Source: CAD feature listing. Evaluate the final solid. Frame: model axes, mm. A direction names the side the tool comes from. Coordinates: 2 decimals unless noted, no trailing zeros. Loops run counter-clockwise (first coordinate to the right, second up) from the corner with the lowest first, then second, coordinate; pieces in that order, holes last. Notation, with made-up numbers: M 81.25,-4.5 L 88.25,-4.5 A16 cw 88.25,10.5 Z; hole C -30.75,1.5 d2. An arc over 180 degrees is marked long. Write each question's results on one line, items separated by ' | '. Start each with the question number.
from build123d import *

# Parameters (mm, degrees)
BOSS_EXTRUDE1_DEPTH = 175


with BuildPart() as part:
    # Sketch1 → Boss-Extrude1 (new body, symmetric)
    with BuildSketch(Plane.XY):
        Polygon((-3.1, 10), (-3.1, 8.200660172), (-5.5, 8.200660172), (-5.5, 6.560660172), (-2.84, 3.900660172), (2.84, 3.900660172), (5.5, 6.560660172), (5.5, 8.200660172), (3.1, 8.200660172), (3.1, 10), (10, 10), (10, 3.1), (8.200660172, 3.1), (8.200660172, 5.5), (6.560660172, 5.5), (3.900660172, 2.84), (3.900660172, -2.84), (6.560660172, -5.5), (8.200660172, -5.5), (8.200660172, -3.1), (10, -3.1), (10, -10), (3.1, -10), (3.1, -8.200660172), (5.5, -8.200660172), (5.5, -6.560660172), (2.84, -3.900660172), (-2.84, -3.900660172), (-5.5, -6.560660172), (-5.5, -8.200660172), (-3.1, -8.200660172), (-3.1, -10), (-10, -10), (-10, -3.1), (-8.200660172, -3.1), (-8.200660172, -5.5), (-6.560660172, -5.5), (-3.900660172, -2.84), (-3.900660172, 2.84), (-6.560660172, 5.5), (-8.200660172, 5.5), (-8.200660172, 3.1), (-10, 3.1), (-10, 10), align=None)
    extrude(amount=BOSS_EXTRUDE1_DEPTH, both=True)


solid = part.part
Item 1: Cut plane A-A (y = 0). Output: boundary loops of the cut face in (x, z), then the cut area to 3 significant figures.
Item 2: Access query for faces 4 (the flat face through (10, 7, 2)), 5 (the flat face through (0, -3.901, 2)), 6 (the flat face through (0, 3.901, 2)), 7 (the flat face through (-7, 10, 2)), 8 (the flat face through (-3.901, 0, 2)). Directions: +Z, -Z, +X, -X, +Y, -Y. A direction counts if a zero-diameter tool reaches every point of the face in a straight line with its end or side. Return the directions, or none.
Item 3: Line query: probe 1 along Y at (x, z) = (-8, 28.5); probe 2 along Y at (x, z) = (9.25, 122.5); probe 3 along Y at (x, z) = (-3.25, 158.5). Output: solid intervals per line, ascending.
Item 4: Mould query, pull axis Y, two halves, no side actions, for faces 1 (the flat face through (7, -10, 2)), 2 (the flat face through (10, -7, 2)), 3 (the flat face through (3.901, 0, 2)). Classes: +Y half, -Y half, draft (parallel to the pull), parting line (faces both ways), or undercut.
Item 5: First-contact query: pin 1 Ø3 at (y, z) = (-1.5, -59.5) entering from -X; pin 2 Ø1.5 at (y, z) = (-2, 82) entering from -X; pin 3 Ø2 at (x, z) = (0, 138) entering from +Y. Flat tips, straight axial feed; report the tip coordinate or a pass-through.
Response values:
1) outline: M -3.9,-175 L 3.9,-175 L 3.9,175 L -3.9,175 Z | area: 2,730 mm2
2) face 4: +Z, -Z, +X, +Y, -Y | face 5: +Z, -Z, -Y | face 6: +Z, -Z, +Y | face 7: +Z, -Z, +X, -X, +Y | face 8: +Z, -Z, -X
3) probe 1: y = -10 to -5.5, 5.5 to 10 | probe 2: y = -10 to -3.1, 3.1 to 10 | probe 3: y = -10 to -8.2, -4.31 to 4.31, 8.2 to 10
4) face 1: -Y half | face 2: draft | face 3: undercut
5) pin 1: stops at x = -4.06 | pin 2: stops at x = -3.9 | pin 3: stops at y = 3.9
